from build123d import *

# Parameters (mm, degrees)
SKETCH1_W                 = 125
SKETCH1_H                 = 130
BOSS_EXTRUDE1_DEPTH       = 22
M5X0_8_TAPPED_HOLE1_D     = 4.2
M5X0_8_TAPPED_HOLE1_DEPTH = 14
M5X0_8_TAPPED_HOLE1_TIP   = 1.2618073


with BuildPart() as part:
    # Sketch1 → Boss-Extrude1 (new body)
    with BuildSketch(Plane.XY):
        with Locations((0, 65)):
            Rectangle(SKETCH1_W, SKETCH1_H)
    extrude(amount=-BOSS_EXTRUDE1_DEPTH)

    # Sketch2 → Cut-Revolve1 (revolve, cut)
    with BuildSketch(Plane(origin=(0, 0, 0), x_dir=(0, 0, -1), z_dir=(1, 0, 0)), mode=Mode.PRIVATE) as cut_revolve1_sk:
        Polygon((0, 109.7), (15, 109.7), (15, 101.2), (22, 101.2), (22, 83.7), (0, 83.7), align=None)
    revolve(cut_revolve1_sk.sketch.rotate(Axis((0, 83.7, 6.088066236), (0, 0, -1)), 90), axis=Axis((0, 83.7, 6.088066236), (0, 0, -1)), mode=Mode.SUBTRACT)

    # M5x0.8 Tapped Hole1
    with Locations(Plane.XZ):
        with Locations((-50, -11), (50, -11)):
            Hole(M5X0_8_TAPPED_HOLE1_D / 2, depth=M5X0_8_TAPPED_HOLE1_DEPTH)
            with Locations((0, 0, -(M5X0_8_TAPPED_HOLE1_DEPTH + M5X0_8_TAPPED_HOLE1_TIP / 2))):  # 118° drill point
                Cone(0, M5X0_8_TAPPED_HOLE1_D / 2, M5X0_8_TAPPED_HOLE1_TIP, mode=Mode.SUBTRACT)


solid = part.part
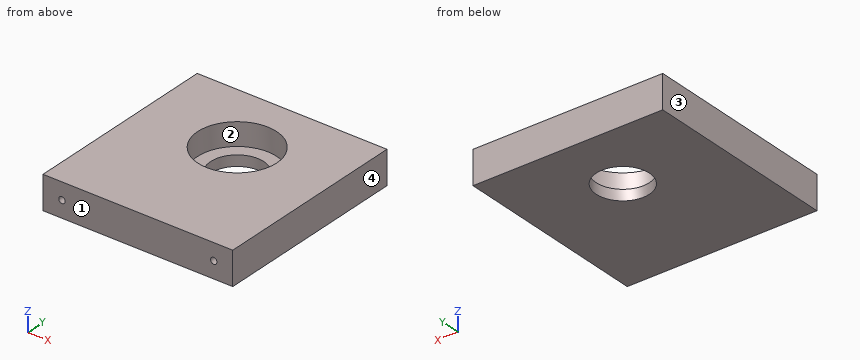
Here's how the part is built. I have some questions about the finished solid (model axes, mm). Face numbers are marked on the shaded views. Give positions to 0.01 mm unless a question says otherwise; leave off trailing zeros. Order: outer loops, then holes, each group sorted by start corner. A loop starts at its lowest first (then second) coordinate and runs counter-clockwise, first axis right, second up. Notation, with made-up numbers: (44, -11) -> (70, -11) arc R24 cw to (70, 3) -> close; hole circle Ø11 at (-28.5, 15.25). An arc over 180 degrees is marked (long way). One line per item, written item: value. Start each with the question number.
1. Imagine slicing it at B-B, the plane y = 96.5. List the corners of the cut face in (x, z) for me.
2. Imagine slicing it at C-C, the plane z = -19.75. List the corners of the cut face in (x, y) for me.
3. Imagine slicing it at D-D, the plane y = 62.5. List the corners of the cut face in (x, z) for me, plus the area to 3 significant figures.
4. Imagine slicing it at A-A, the plane x = 0. List the corners of the cut face in (y, z) for me, plus the area to 4 significant figures.
5. We'd pull the mould along X, two halves only. Please class the marked faces 1, 2, 3 and 4: released by +X, released by -X, zero draft, split by the parting line, or undercut.
6. I need wall thicknesses on probe 1 along X at (y, z) = (5.75, -11); probe 2 along X at (y, z) = (83.7, -18.5); probe 3 along Z at (x, y) = (-50, 7.25). Which ranges of each line are inside material? Lowest first, please. Write a range as from..to.
Values follow:
1. outline: (-62.5, -22) -> (-11.93, -22) -> (-11.93, -15) -> (-22.63, -15) -> (-22.63, 0) -> (-62.5, 0) -> close; (11.93, -22) -> (62.5, -22) -> (62.5, 0) -> (22.63, 0) -> (22.63, -15) -> (11.93, -15) -> close
2. outline: (-62.5, 0) -> (62.5, 0) -> (62.5, 130) -> (-62.5, 130) -> close; hole circle Ø35 at (0, 83.7)
3. outline: (-62.5, -22) -> (62.5, -22) -> (62.5, 0) -> (15.05, 0) -> (15.05, -15) -> (-15.05, -15) -> (-15.05, 0) -> (-62.5, 0) -> close
3. area: 2,300 mm2
4. outline: (0, -22) -> (66.2, -22) -> (66.2, -15) -> (57.7, -15) -> (57.7, 0) -> (0, 0) -> close; (101.2, -22) -> (130, -22) -> (130, 0) -> (109.7, 0) -> (109.7, -15) -> (101.2, -15) -> close
4. area: 1,835 mm2
5. face 1: zero draft
5. face 2: undercut
5. face 3: released by -X
5. face 4: released by +X
6. probe 1: x = -62.5..-52.1, -47.9..47.9, 52.1..62.5
6. probe 2: x = -62.5..-17.5, 17.5..62.5
6. probe 3: z = -22..-13.1, -8.9..0
